```python
from build123d import *

# Parameters (mm, degrees)
SKETCH1_W                = 28
SKETCH1_H                = 35
SKETCH1_R                = 3.05
BOSS_EXTRUDE1_DEPTH      = 40
CUT_EXTRUDE1_DEPTH       = 46.85029989
CUT_EXTRUDE1_DEPTH_BACK  = 46.85029989
SKETCH2_R                = 5
BOSS_EXTRUDE2_DEPTH      = 5
BOSS_EXTRUDE2_DEPTH_BACK = 5
SKETCH4_W                = 210
SKETCH4_H                = 35
FILLET1_R                = 10


with BuildPart() as part:
    # Sketch1 → Boss-Extrude1 (new body)
    with BuildSketch(Plane.XY):
        Rectangle(SKETCH1_W, SKETCH1_H)
        Circle(SKETCH1_R, mode=Mode.SUBTRACT)
    extrude(amount=-BOSS_EXTRUDE1_DEPTH)

    # Sketch2 → Cut-Extrude1 (cut, two sides: drawn at the far end of the back side and taken through both)
    with BuildSketch(Plane(origin=(0, 0, 0), x_dir=(0, 0, -1), z_dir=(1, 0, 0)).offset(-CUT_EXTRUDE1_DEPTH_BACK)):
        with Locations((20, 0)):
            Circle(SKETCH2_R)
    extrude(amount=CUT_EXTRUDE1_DEPTH + CUT_EXTRUDE1_DEPTH_BACK, mode=Mode.SUBTRACT)

    # Sketch4 → Boss-Extrude2 (add, two sides: drawn at the far end of the back side and taken through both)
    with BuildSketch(Plane(origin=(0, 0, 0), x_dir=(0, 0, -1), z_dir=(1, 0, 0)).offset(-BOSS_EXTRUDE2_DEPTH_BACK)):
        with Locations((145, 0)):
            Rectangle(SKETCH4_W, SKETCH4_H)
        with BuildLine():
            Line((235, -6), (155, -6))
            ThreePointArc((155, -6), (149, 0), (155, 6))
            Line((155, 6), (235, 6))
            ThreePointArc((235, 6), (241, 0), (235, -6))
        make_face(mode=Mode.SUBTRACT)
    extrude(amount=BOSS_EXTRUDE2_DEPTH + BOSS_EXTRUDE2_DEPTH_BACK)

    # Fillet1
    fillet1_edges = [part.edges().sort_by_distance(p)[0] for p in [
        (0, 17.5, -250),
        (0, -17.5, -250),
    ]]
    fillet(fillet1_edges, radius=FILLET1_R)


solid = part.part
```
Here's how the part is built. I have some questions about the finished solid (model axes, mm). A direction names the side the tool comes from. Give positions to 0.01 mm unless a question says otherwise; leave off trailing zeros. Order: outer loops, then holes, each group sorted by start corner. A loop starts at its lowest first (then second) coordinate and runs counter-clockwise, first axis right, second up. Notation, with made-up numbers: M -3.75,-11 L 54.25,-11 A20 ccw 54.25,6 Z; hole C -13.5,15.5 d6. An arc over 180 degrees is marked long. Use a Markdown table: item, result. Add a question column.
1. I need wall thicknesses on probe 1 along Y at (x, z) = (0, -34.25); probe 2 along X at (y, z) = (0, -6.75); probe 3 along Y at (x, z) = (-3.5, -179.5). Which ranges of each line are inside material? Lowest first, please. Write a range as from..to.
2. Suppose I cut it at C-C (y = 0). List the corners of the cut face in (x, z) for me, and give its area (3 significant figures).
3. On a 3-axis mill with a long thin cutter (end or side, diameter ignored), from which of +Z, -Z, +X, -X, +Y, -Y can I reach the whole of each face in a straight line? I mean faces 1 (the flat face through (5, 0, -144)), 2 (the cylindrical face through (0, 0, -241)), 3 (the flat face through (0, 17.5, -92)), 4 (the flat face through (-10, 0, -40)), 5 (the flat face through (0, 0, -40)). Say none if no direction works.
4. Suppose I cut it at D-D (z = -105). List the corners of the cut face in (x, y) for me.
5. Suppose I cut it at B-B (x = 0). List the corners of the cut face in (y, z) for me.
6. Suppose I cut it at A-A (z = -212.5). List the corners of the cut face in (x, y) for me.
7. If we mould it in two halves opening along X, with no side actions, what happens to faces 6 (the flat face through (-5, 0, -144)), 7 (the cylindrical face through (2.91, 0.92, -7.91)), 8 (the flat face through (0, -6, -196))? For each: +X half, -X half, draft (parallel to the pull), parting line (faces both ways), or undercut.
8. For pin 1 Ø2.5 at (x, y) = (-11.5, -6.5) entering from -Z; pin 2 Ø17.5 at (y, z) = (5.5, -191) entering from +X; pin 3 Ø17.5 at (y, z) = (8, -164) entering from -X; pin 4 Ø6 at (y, z) = (0, -20) entering from -X, each with a flat end and sliding along its axis, tell me the tip position at first contact or that it passes through.
Results list:
| question | item | result |
|---|---|---|
| 1 | probe 1 | y = -17.5..-3.05, 3.05..17.5 |
| 1 | probe 2 | x = -14..-3.05, 3.05..14 |
| 1 | probe 3 | y = -17.5..-6, 6..17.5 |
| 2 | outline | M -14,-40 L -5,-40 L -5,-149 L 5,-149 L 5,-40 L 14,-40 L 14,-25 L 3.05,-25 L 3.05,-40 L -3.05,-40 L -3.05,-25 L -14,-25 Z; M -14,-15 L -3.05,-15 L -3.05,0 L -14,0 Z; M -5,-250 L 5,-250 L 5,-241 L -5,-241 Z; M 3.05,-15 L 14,-15 L 14,0 L 3.05,0 Z |
| 2 | area | 1,840 mm² |
| 3 | face 1 | -Z, +X, +Y, -Y |
| 3 | face 2 | +X, -X |
| 3 | face 3 | +Z, -Z, +X, -X, +Y |
| 3 | face 4 | -Z, -X, +Y, -Y |
| 3 | face 5 | +Z |
| 4 | outline | M -5,-17.5 L 5,-17.5 L 5,17.5 L -5,17.5 Z |
| 5 | outline | M -17.5,-240 A10 ccw -7.5,-250 L 7.5,-250 A10 ccw 17.5,-240 L 17.5,0 L 3.05,0 L 3.05,-16.04 A5 cw 3.05,-23.96 L 3.05,-40 L -3.05,-40 L -3.05,-23.96 A5 cw -3.05,-16.04 L -3.05,0 L -17.5,0 Z; hole M -6,-235 A6 ccw 6,-235 L 6,-155 A6 ccw -6,-155 Z |
| 6 | outline | M -5,-17.5 L 5,-17.5 L 5,-6 L -5,-6 Z; M -5,6 L 5,6 L 5,17.5 L -5,17.5 Z |
| 7 | face 6 | -X half |
| 7 | face 7 | undercut |
| 7 | face 8 | draft |
| 8 | pin 1 | stops at z = -40 |
| 8 | pin 2 | stops at x = 5 |
| 8 | pin 3 | stops at x = -5 |
| 8 | pin 4 | passes through |
